from build123d import *

# Parameters (mm, degrees)
BOSS_EXTRUDE1_DEPTH = 67.5
BOSS_EXTRUDE2_START = 67.5
SKETCH1_3_R         = 4.425
BOSS_EXTRUDE2_DEPTH = 12.5
BOSS_EXTRUDE4_DEPTH = 11


with BuildPart() as part:
    # Sketch1 → Boss-Extrude1 (new body, symmetric)
    with BuildSketch(Plane(origin=(0, 0, 0), x_dir=(0, 0, -1), z_dir=(1, 0, 0))):
        Polygon((3.75, 0), (1.875, 3.247595264), (-1.875, 3.247595264), (-3.75, 0), (-1.875, -3.247595264), (1.875, -3.247595264), align=None)
    extrude(amount=BOSS_EXTRUDE1_DEPTH, both=True)

    # Sketch1_3 → Boss-Extrude2 (add)
    with BuildSketch(Plane(origin=(0, 0, 0), x_dir=(0, 0, -1), z_dir=(1, 0, 0)).offset(BOSS_EXTRUDE2_START)):
        Circle(SKETCH1_3_R)
    boss_extrude2 = extrude(amount=BOSS_EXTRUDE2_DEPTH)

    # Sketch4 → Boss-Extrude4 (add)
    with BuildSketch(Plane(origin=(80, 0, 0), x_dir=(0, 0, -1), z_dir=(1, 0, 0))):
        with BuildLine():
            Line((1.303840481, 1.45), (-1.303840481, 1.45))
            ThreePointArc((-1.303840481, 1.45), (-0.793728878, -1.78114976), (1.95, 0))
            ThreePointArc((1.95, 0), (1.78114976, 0.793728878), (1.303840481, 1.45))
        make_face()
    boss_extrude4 = extrude(amount=BOSS_EXTRUDE4_DEPTH)

    # Mirror2: Boss-Extrude2, Boss-Extrude4 across plane
    add(boss_extrude2.mirror(Plane(origin=(0, 0, 0), x_dir=(0, 0, 1), z_dir=(1, 0, 0))))
    add(boss_extrude4.mirror(Plane(origin=(0, 0, 0), x_dir=(0, 0, 1), z_dir=(1, 0, 0))))


solid = part.part
The model under review builds one solid part; all positions refer to its coordinate system, in mm. A direction names the side the tool comes from. Round coordinates to 2 decimals unless told otherwise and drop trailing zeros. Order: outer loops, then holes, each group sorted by start corner. A loop starts at its lowest first (then second) coordinate and runs counter-clockwise, first axis right, second up. Notation, with made-up numbers: (33, 48) -> (62, 48) arc R19 ccw to (62, 56) -> close; hole circle Ø1 at (-15.75, 59.5). An arc over 180 degrees is marked (long way). Use CSV: the item, a comma, the result in double quotes. Start each with the question number.
(1) Insertion check: pin 1 (0.8 mm diameter, centred on x = 88, z = -0.5, fed in from +Y); pin 2 (1.9 mm diameter, centred on x = 21, z = -0.5, fed in from -Y); pin 3 (4 mm diameter, centred on x = 19, z = -0.5, fed in from +Y). Each pin has a flat end and moves straight along its axis. Give the tip position at first contact, or say it passes through.
(2) Wall thickness on probe 1 along X at (y, z) = (-3.5, -1); probe 2 along X at (y, z) = (-2.75, 1.5); probe 3 along Y at (x, z) = (7, 0): over which ranges is each line inside the solid? List them lowest first. Write a range as from..to.
(3) Consider section A-A on x = -48. Write out the cut boundary in (y, z) (3 decimals).
(4) Tool access review of faces 1 (the face through (0.945, -1.601, 2.826)), 2 (the face through (-80, -1, -2)), 3 (the face through (1, 3.248, 0)), 4 (the face through (80, -1, -2)): name each direction out of +Z, -Z, +X, -X, +Y, -Y from which nothing blocks a thin tool from reaching the whole face with its end or side.
Responses:
1,pin 1,"y = 1.45"
1,pin 2,"y = -3.25"
1,pin 3,"y = 3.25"
2,probe 1,"-80..-67.5, 67.5..80"
2,probe 2,"-80..80"
2,probe 3,"-3.25..3.25"
3,outline,"(-3.248, -1.875) -> (0, -3.75) -> (3.248, -1.875) -> (3.248, 1.875) -> (0, 3.75) -> (-3.248, 1.875) -> close"
4,face 1,"+Z, -Y"
4,face 2,"-X"
4,face 3,"+Z, -Z, +Y"
4,face 4,"+X"
